Can you work these out from the model? Positions are in its coordinate system, mm. Coordinates: 2 decimals unless noted, no trailing zeros. Order: outer loops, then holes, each group sorted by start corner. A loop starts at its lowest first (then second) coordinate and runs counter-clockwise, first axis right, second up. Notation, with made-up numbers: (-14.75, 52.25) -> (18.25, 52.25) arc R7 cw to (18.25, 59.25) -> close; hole circle Ø9 at (6, 24). An arc over 180 degrees is marked (long way). Answer in a Markdown table with one row per item. Add a question column.
1. Imagine slicing it at B-B on y = 5847.5. Write out the boundary of the cut face in (x, z).
2. Imagine slicing it at A-A on z = 40168. Write out the boundary of the cut face in (x, y), plus the area to 3 significant figures.
3. Imagine slicing it at D-D on z = 39980. Write out the boundary of the cut face in (x, y), plus the area to 3 significant figures.
4. Will this pin go through, and if not, where does the flat tip stop? pin 1 (1 mm diameter, centred on y = 5848, z = 39962.5, fed in from +X).
5. Imagine slicing it at C-C on x = -22901. Write out the boundary of the cut face in (y, z).
6. If I drill on line 1 along Z through (x, y) = (-23012, 5856.25); line 2 along X through (y, z) = (5852.25, 40135.5); line 3 along X through (y, z) = (5851.25, 39940), over which ranges is the centre line in solid material (lowest first)? Write a range as [from, to].
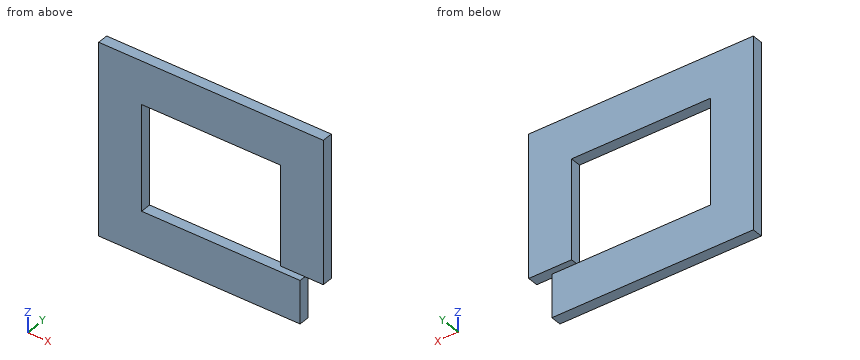
from build123d import *

# Parameters (mm, degrees)
BOSS_EXTRUDE1_START = 550
SKETCH1_W           = 80
SKETCH1_H           = 276.203950277
SKETCH1_W_2         = 295.879209743
SKETCH1_H_2         = 80
SKETCH1_H_3         = 12.7
BOSS_EXTRUDE1_DEPTH = 20


with BuildPart() as part:
    # Sketch1 → Boss-Extrude1 (new body)
    with BuildSketch(Plane(origin=(0, 5294.457128547, 0), x_dir=(1, 0, 0), z_dir=(0, 1, 0)).offset(BOSS_EXTRUDE1_START)):
        with Locations((-23153.790093454, -40062.769337853)):
            Rectangle(SKETCH1_W, SKETCH1_H)
        Polygon((-23113.790093454, -40200.871312991), (-23193.790093454, -40200.871312991), (-23193.790093454, -40280.871312991), (-22854.669978064, -40280.871312991), (-22854.669978064, -40200.871312991), align=None)
        Polygon((-22854.669978064, -40028.167362714), (-22854.669978064, -40200.871312991), (-22854.669978064, -40280.871312991), (-22774.669978064, -40280.871312991), (-22774.669978064, -40028.167362714), align=None)
        with Locations((-22965.850488583, -39964.667362714)):
            Rectangle(SKETCH1_W_2, SKETCH1_H_2)
        with Locations((-22814.669978064, -40021.817362714)):
            Rectangle(SKETCH1_W, SKETCH1_H_3)
    extrude(amount=BOSS_EXTRUDE1_DEPTH)


solid = part.part
Answers follow:
| question | item | result |
|---|---|---|
| 1 | outline | (-23193.79, 39924.67) -> (-22817.91, 39924.67) -> (-22817.91, 40004.67) -> (-23113.79, 40004.67) -> (-23113.79, 40200.87) -> (-22854.67, 40200.87) -> (-22854.67, 40015.47) -> (-22774.67, 40015.47) -> (-22774.67, 40280.87) -> (-23193.79, 40280.87) -> close |
| 2 | outline | (-23193.79, 5844.46) -> (-23113.79, 5844.46) -> (-23113.79, 5864.46) -> (-23193.79, 5864.46) -> close; (-22854.67, 5844.46) -> (-22774.67, 5844.46) -> (-22774.67, 5864.46) -> (-22854.67, 5864.46) -> close |
| 2 | area | 3,200 mm² |
| 3 | outline | (-23193.79, 5844.46) -> (-22817.91, 5844.46) -> (-22817.91, 5864.46) -> (-23193.79, 5864.46) -> close |
| 3 | area | 7,520 mm² |
| 4 | pin 1 | stops at x = -22817.91 |
| 5 | outline | (5844.46, 39924.67) -> (5864.46, 39924.67) -> (5864.46, 40004.67) -> (5844.46, 40004.67) -> close; (5844.46, 40200.87) -> (5864.46, 40200.87) -> (5864.46, 40280.87) -> (5844.46, 40280.87) -> close |
| 6 | line 1 | z = [39924.67, 40004.67], [40200.87, 40280.87] |
| 6 | line 2 | x = [-23193.79, -23113.79], [-22854.67, -22774.67] |
| 6 | line 3 | x = [-23193.79, -22817.91] |
